```python
from build123d import *

# Parameters (mm, degrees)
F2_R     = 71.4411374157
F3_DEPTH = 5
F4_R     = 71.0302069346
F6_DEPTH = 25
F7_R     = 0.0241421356


# Not quite as in the source:
# - a fillet or chamfer that OpenCascade refuses, or shapes differently, is made with other operations: its cross-section is extruded or revolved along the edge and cut away or added


with BuildPart() as f3:
    # F2 (on Top) → F3 (new body)
    with BuildSketch(Plane.XY):
        Circle(F2_R)
    extrude(amount=F3_DEPTH)

    # F4 (on face) → F6 (join)
    with BuildSketch(Plane(origin=(0, 0, 0), x_dir=(1, 0, 0), z_dir=(0, 0, -1))):
        Circle(F4_R)
    extrude(amount=F6_DEPTH)

    # F7
    f7_edges = [f3.edges().sort_by_distance(p)[0] for p in [
        (-71.441137, 0, 0),
    ]]
    fillet(f7_edges, radius=F7_R)

    # F8: chamfer of 5 on 1 edges, made by hand

    # F8_s1 → F8_t2 (revolve, cut)
    with BuildSketch(Plane.XZ):
        Polygon((71.4411374157, 0), (66.4411374157, 5), (71.4411374157, 5), align=None)
    revolve(axis=Axis((0, 0, 5), (0, 0, 1)), mode=Mode.SUBTRACT)

    # F9: fillet of radius 5 on 3 edges, made by hand

    # F9_s1 → F9_t2 (revolve, cut)
    with BuildSketch(Plane.XZ):
        with BuildLine():
            ThreePointArc((71.0302069346, -20), (69.5657408405, -23.5355339059), (66.0302069346, -25))
            Line((66.0302069346, -25), (66.0302069346, -25.1))
            Line((66.0302069346, -25.1), (71.1302069346, -25.1))
            Line((71.1302069346, -25.1), (71.1302069346, -20))
            Line((71.1302069346, -20), (71.0302069346, -20))
        make_face()
    revolve(axis=Axis((0, 0, -25), (0, 0, -1)), mode=Mode.SUBTRACT)

    # F9_s3 → F9_t4 (revolve)
    with BuildSketch(Plane.XZ):
        with BuildLine():
            ThreePointArc((71.4340663479, 0.0070710678), (71.1322122973, -0.9567431048), (71.0302069346, -1.9615557905))
            Line((71.0302069346, -1.9615557905), (70.9302069346, -1.9615557905))
            Line((70.9302069346, -1.9615557905), (70.9302069346, 0))
            Line((70.9302069346, 0), (71.0302069346, 0.1))
            ThreePointArc((71.0302069346, 0.1), (71.2321366412, 0.1), (71.3421435362, 0.046443605))
            Line((71.3421435362, 0.046443605), (71.4340663479, 0.0070710678))
        make_face()
    revolve(axis=Axis((0, 0, 0), (0, 0, -1)))


solid = f3.part
```
The listing builds one solid part. Answer for the finished solid, in the listing's coordinates (mm). A direction names the side the tool comes from. Coordinates: 2 decimals unless noted, no trailing zeros. Write each loop counter-clockwise with the first axis right and the second up, starting at its lowest first coordinate (ties: lowest second). Pieces come first, ordered by that corner, then holes. Notation, with made-up numbers: (-18.5, 25) - (-12.5, 25) arc R22 cw to (-12.5, 64) - close; hole circle Ø11 at (-3.5, -1.75). An arc over 180 degrees is marked (long way). Return JSON: item names as keys, results as strings. Group by question number.
Q1. The part is cut by section A-A on z = -9.5. Write down the section's boundary in (x, y), and give its area (3 significant figures).
Q2. Flat-ended cylindrical pins translate along their axes: pin 1 Ø8 at (x, z) = (1.5, 1) entering from +Y; pin 2 Ø3 at (x, z) = (13.5, -14.5) entering from +Y; pin 3 Ø1 at (x, z) = (44.5, -14) entering from -Y. Find the tip coordinate at first contact, or state that the pin passes through.
Q3. The part is cut by section B-B on z = -22.75. Write down the section's boundary in (x, y).
Q4. Which of the six approach directions +Z, -Z, +X, -X, +Y, -Y give full straight-line access (tool end or side, diameter ignored) to faces 1 (the conical face through (-52.918, -40.576, 4.758)), 2 (the cylindrical face through (-15.4, 69.34, -10.85))?
Q5. Find the intervals of material crossed by line 1 along X through (y, z) = (-18.5, -3); line 2 along Y through (x, z) = (19, -21.25); line 3 along X through (y, z) = (16, -20.5), in increasing order. Write a range as [from, to].
Evaluation:
{
 "1": {"outline": "circle Ø142.06 at (0, 0)", "area": "15,900 mm2"},
 "2": {"pin 1": "stops at y = 71.43", "pin 2": "stops at y = 70.01", "pin 3": "stops at y = -55.76"},
 "3": {"outline": "circle Ø140.41 at (0, 0)"},
 "4": {"face 1": "+Z", "face 2": "-Z"},
 "5": {"line 1": "x = [-68.58, 68.58]", "line 2": "y = [-68.28, 68.28]", "line 3": "x = [-69.18, 69.18]"}
}
